```python
from build123d import *

# Parameters (mm, degrees)
F0_W          = 88.9
F0_H          = 88.9
F1_DEPTH      = 863.6
F2_W          = 513.853363
F2_H          = 520.7
F3_DEPTH      = 88.9
F6_W          = 475.753363
F6_H          = 482.6
F7_DEPTH      = 88.9
F9_DEPTH      = 18.796
F9_DEPTH_BACK = 0.254
F10_W         = 801.376414
F10_H         = 19.05
F10_W_2       = 19.05
F10_H_2       = 381
F11_DEPTH     = 743.204


with BuildPart() as f1:
    # F0 (on Top) → F1 (new body)
    with BuildSketch(Plane.XY):
        Polygon((-26.038207, -26.038207), (-88.9, -88.9), (-26.038207, -151.761793), (36.823586, -88.9), (125.723586, -88.9), (125.723586, 0), (36.823586, 0), (0, 0), align=None)
        with Locations((971.55, -44.45)):
            Rectangle(F0_W, F0_H)
        Polygon((-511.874599, -511.874599), (-574.736392, -574.736392), (-511.874599, -637.598185), (-449.012806, -574.736392), align=None)
        Polygon((-170.624866, -978.847917), (-107.763073, -1041.70971), (-44.901281, -978.847917), (-107.763073, -915.986124), align=None)
        Polygon((312.284844, -621.661793), (375.146637, -558.8), (464.046637, -558.8), (464.046637, -469.9), (375.146637, -469.9), (338.323051, -469.9), (312.284844, -495.938207), (249.423051, -558.8), align=None)
        with Locations((971.55, -514.35)):
            Rectangle(F0_W, F0_H)
    extrude(amount=-F1_DEPTH)


with BuildPart() as f3:
    # F2 (on Top) → F3 (new body)
    with BuildSketch(Plane.XY):
        Polygon((1016, 0), (0, 0), (-574.736392, -574.736392), (-107.763073, -1041.70971), (375.146637, -558.8), (1016, -558.8), align=None)
        Polygon((367.255868, -539.75), (-107.763073, -1014.768942), (-547.795623, -574.736392), (7.890768, -19.05), (464.046637, -19.05), (464.046637, -539.75), align=None, mode=Mode.SUBTRACT)
        with Locations((740.023318, -279.4)):
            Rectangle(F2_W, F2_H, mode=Mode.SUBTRACT)
    extrude(amount=-F3_DEPTH)


with BuildPart() as f1_1:
    add(f1.part)

    # F4: union F3
    add(f3.part)

    # F6 (on offset) → F7 (join)
    with BuildSketch(Plane.XY.offset(-762)):
        Polygon((1016, 0), (0, 0), (-574.736392, -574.736392), (-107.763073, -1041.70971), (375.146637, -558.8), (1016, -558.8), align=None)
        Polygon((-107.763073, -987.828173), (-520.854855, -574.736392), (-154.688475, -208.570011), (258.403307, -621.661793), align=None, mode=Mode.SUBTRACT)
        Polygon((-127.747706, -181.629243), (15.781537, -38.1), (464.046637, -38.1), (464.046637, -520.7), (359.3651, -520.7), (285.344075, -594.721024), align=None, mode=Mode.SUBTRACT)
        with Locations((740.023318, -279.4)):
            Rectangle(F6_W, F6_H, mode=Mode.SUBTRACT)
    extrude(amount=-F7_DEPTH)

    # F8 (on face) → F9 (join, two sides)
    with BuildSketch(Plane.XY.offset(-762)) as f9_sk:
        Polygon((-574.736392, -574.736392), (-107.763073, -1041.70971), (375.146637, -558.8), (1016, -558.8), (1016, 0), (0, 0), align=None)
    extrude(amount=F9_DEPTH)
    extrude(f9_sk.sketch, amount=-F9_DEPTH_BACK)

    # F10 (on Top) → F11 (join, through all)
    with BuildSketch(Plane.XY):
        with Locations((526.411793, -28.575)):
            Rectangle(F10_W, F10_H)
        with Locations((987.425, -279.4)):
            Rectangle(F10_W_2, F10_H_2)
        Polygon((44.374324, -83.093798), (29.272848, -94.706202), (326.710647, -481.512404), (341.812123, -469.9), align=None)
        Polygon((-484.933831, -610.657416), (-498.404215, -624.1278), (-157.154482, -965.377533), (-143.684098, -951.907149), align=None)
    extrude(amount=-F11_DEPTH)


solid = f1_1.part
```
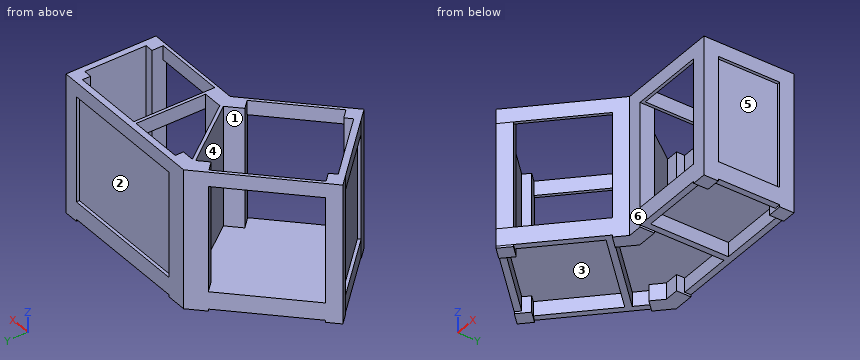
Geometry check sheet. Reference: the model listing, model coordinates, mm. Face numbers are marked on the shaded views. A direction names the side the tool comes from. Give positions to 0.01 mm unless a question says otherwise; leave off trailing zeros. Loops run counter-clockwise (first coordinate to the right, second up) from the corner with the lowest first, then second, coordinate; pieces in that order, holes last. Notation, with made-up numbers: M 4,-27 L 62,-27 A20 ccw 62,8 Z; hole C 40.25,14.5 d7. An arc over 180 degrees is marked long. Write item = value, one per line.
(1) Sectioned sample at A-A, the plane x = 520.5. Record the cut outline in (y, z), plus the area to 3 significant figures.
Answer below:
outline = M -558.8,-850.9 L -520.7,-850.9 L -520.7,-762.25 L -38.1,-762.25 L -38.1,-850.9 L 0,-850.9 L 0,-743.2 L -19.05,-743.2 L -19.05,-88.9 L 0,-88.9 L 0,0 L -38.1,0 L -38.1,-743.2 L -558.8,-743.2 Z; M -558.8,-88.9 L -539.75,-88.9 L -539.75,0 L -558.8,0 Z
area = 34,900 mm2
(2) Sectioned sample at B-B, the plane z = -791.5. State how many separate pieces and enclosed holes the cut face has, plus the area to 3 significant figures.
Answer below:
separate_pieces = 1
enclosed_holes = 3
area = 234,000 mm2
(3) Tool access check on the marked faces 4, 5 and 6. Record the directions out of +Z, -Z, +X, -X, +Y, -Y that give a thin tool (end or side, any length) a straight path to the whole face; none if there is none.
Answer below:
face_4 = +Z
face_5 = +X
face_6 = +Z, -Z, +X, -Y
(4) Material ranges on line 1 (Y direction, x = 300.5, z = -355.5); line 2 (Y direction, x = 309, z = -471.5); line 3 (Z direction, x = -42.5, y = -865), recorded low to high. Write a range as [from, to].
Answer below:
line_1 = [-609.88, -507.72], [-447.43, -416.18], [-38.1, -19.05]
line_2 = [-618.38, -499.22], [-458.48, -427.23], [-38.1, -19.05]
line_3 = [-762.25, -743.2]
(5) Release check for a two-part mould opening along Z. For the marked faces 1, 2 and 3 record: released by +Z, released by -Z, zero draft, split by the parting line, or undercut.
Answer below:
face_1 = zero draft
face_2 = undercut
face_3 = released by -Z
(6) Sectioned sample at C-C, the plane y = -896. Record the cut outline in (x, z).
Answer below:
outline = M -253.47,-850.9 L -199.59,-850.9 L -199.59,-762.25 L -15.93,-762.25 L -15.93,-850.9 L 37.95,-850.9 L 37.95,-743.2 L -199.59,-743.2 L -199.59,0 L -253.47,0 L -253.47,-88.9 L -226.53,-88.9 L -226.53,-743.2 L -253.47,-743.2 Z; M 11.01,-88.9 L 37.95,-88.9 L 37.95,0 L 11.01,0 Z
(7) Gauge pin test, flat ends, axial feed: pin 1 Ø5 at (x, y) = (115.5, -472) entering from +Z; pin 2 Ø10 at (x, z) = (-367.5, -771) entering from -Y; pin 3 Ø4 at (y, z) = (-109, -565.5) entering from +X. Record the tip position at first contact, or that the pin passes through.
Answer below:
pin_1 = -743.2
pin_2 = -786.97
pin_3 = 996.95
(8) Sectioned sample at D-D, the plane x = 88. Record the cut outline in (y, z), plus the area to 3 significant figures.
Answer below:
outline = M -845.95,-850.9 L -792.07,-850.9 L -792.07,-762.25 L -451.26,-762.25 L -451.26,-850.9 L -397.38,-850.9 L -397.38,-762.25 L -88.9,-762.25 L -88.9,-863.6 L 0,-863.6 L 0,0 L -88.9,0 L -88.9,-743.2 L -139.83,-743.2 L -139.83,0 L -171.08,0 L -171.08,-743.2 L -845.95,-743.2 Z; M -845.95,-88.9 L -819.01,-88.9 L -819.01,0 L -845.95,0 Z
area = 126,000 mm2
